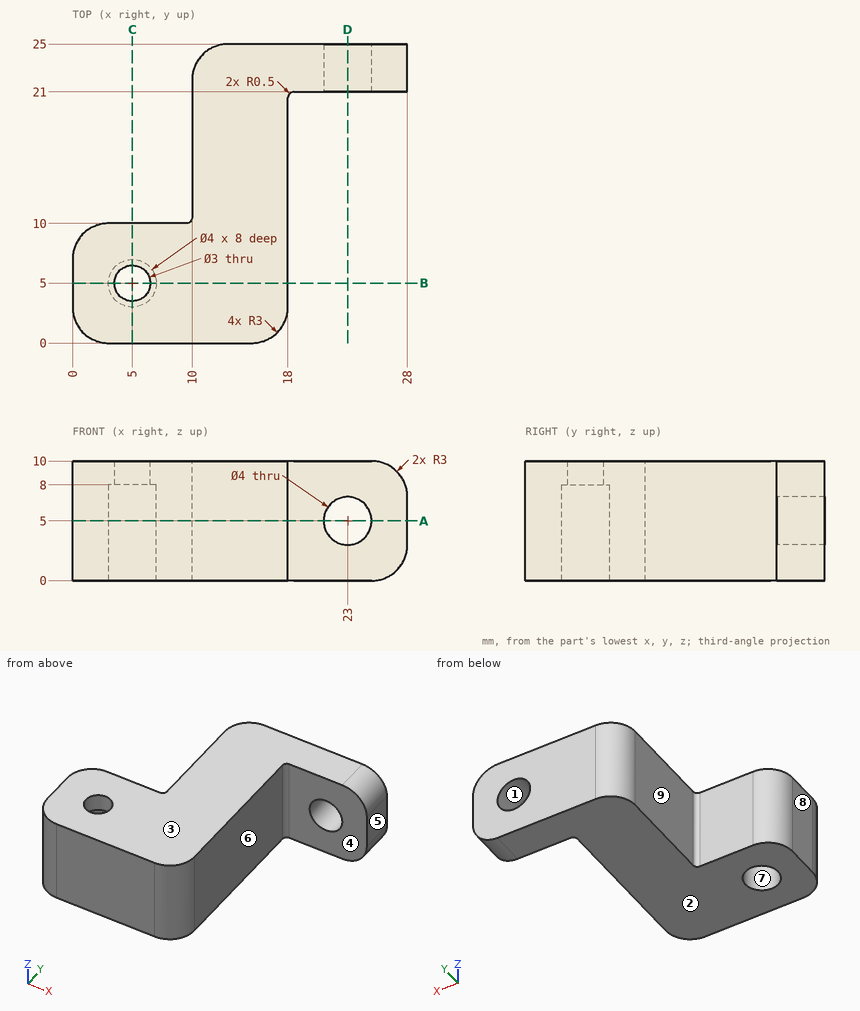
For this review, use the dimensioned drawing (mm, ordinates from the lowest corner) and the shaded views. A direction names the side the tool comes from. Give positions to 0.01 mm unless a question says otherwise; leave off trailing zeros. Write each loop counter-clockwise with the first axis right and the second up, starting at its lowest first coordinate (ties: lowest second). Pieces come first, ordered by that corner, then holes. Notation, with made-up numbers: M -9,34 L 21,34 A10 ccw 21,52 Z; hole C 75.25,-37.5 d3. An arc over 180 degrees is marked long. Write item = value, one per line. Start each with the question number.
Q1. We need section C-C (x = 5). State the section outline as (y, z) points, plus the area to 3 significant figures.
Q2. Machinability: for the marked faces 5, 6, 7, 8 and 9, which of the approach directions +Z, -Z, +X, -X, +Y, -Y give a long, thin tool a straight path to every point of the face, cutting with its end or side? Answer none if there is none.
Q3. We need section B-B (y = 5). State the section outline as (x, z) points.
Q4. Clearance check with flat-ended pins moving along their axes: pin 1 (3 mm diameter, centred on x = 6, z = 7, fed in from +Y); pin 2 (1.5 mm diameter, centred on y = 9.5, z = 8.5, fed in from +X); pin 3 (3 mm diameter, centred on x = 23, z = 5, fed in from +Y); pin 4 (3.5 mm diameter, centred on x = 5, y = 5, fed in from +Z). State where each tip first meets the part, or that it passes through.
Q5. We need section A-A (z = 5). State the section outline as (x, y) points.
Q6. Mouldability with a two-part tool opening along Z and no side actions: class the marked faces 1, 2, 3 and 4 as released by +Z, released by -Z, zero draft, split by the parting line, or undercut.
Q7. For line 1 (Z direction, x = 23, y = 23.8); line 2 (Y direction, x = 5, z = 8.9), list the stretches that pass through material, from the lowest coordinate up.
Q8. We need section D-D (x = 23). State the section outline as (y, z) points.
Result set:
q1.outline = M 0,0 L 3,0 L 3,8 L 3.5,8 L 3.5,10 L 0,10 Z; M 6.5,8 L 7,8 L 7,0 L 10,0 L 10,10 L 6.5,10 Z
q1.area = 62.0 mm2
q2.face_5 = +Z, -Z, +X, +Y, -Y
q2.face_6 = +Z, -Z, +X, -Y
q2.face_7 = -Z
q2.face_8 = +Z, -Z, -X, +Y, -Y
q2.face_9 = +Z, -Z, -X, +Y
q3.outline = M 0,0 L 3,0 L 3,8 L 3.5,8 L 3.5,10 L 0,10 Z; M 6.5,8 L 7,8 L 7,0 L 18,0 L 18,10 L 6.5,10 Z
q4.pin_1 = 10
q4.pin_2 = 18
q4.pin_3 = through
q4.pin_4 = 10
q5.outline = M 0,3 A3 ccw 3,0 L 15,0 A3 ccw 18,3 L 18,20.5 A0.5 cw 18.5,21 L 21,21 L 21,25 L 13,25 A3 ccw 10,22 L 10,10.5 A0.5 cw 9.5,10 L 3,10 A3 ccw 0,7 Z; M 25,21 L 28,21 L 28,25 L 25,25 Z; hole C 5,5 d4
q6.face_1 = undercut
q6.face_2 = released by -Z
q6.face_3 = released by +Z
q6.face_4 = zero draft
q7.line_1 = 0 to 3, 7 to 10
q7.line_2 = 0 to 3.5, 6.5 to 10
q8.outline = M 21,0 L 25,0 L 25,3 L 21,3 Z; M 21,7 L 25,7 L 25,10 L 21,10 Z
